The model under review builds one solid part; all positions refer to its coordinate system, in mm. Face numbers are marked on the shaded views. A direction names the side the tool comes from. Give positions to 0.01 mm unless a question says otherwise; leave off trailing zeros. Order: outer loops, then holes, each group sorted by start corner. A loop starts at its lowest first (then second) coordinate and runs counter-clockwise, first axis right, second up. Notation, with made-up numbers: (12, 74) - (69, 74) arc R21 cw to (69, 107) - close; hole circle Ø9 at (24, -38). An arc over 180 degrees is marked (long way). Use CSV: the item, a comma, the result in double quotes.
```python
from build123d import *

# Parameters (mm, degrees)
F1_DEPTH  = 44
F3_DEPTH  = 45.2
F4_DEPTH  = 52
F5_R      = 4
F6_DEPTH  = 57.3
F7_R      = 7.25
F8_DEPTH  = 25
F9_R      = 3
F10_R     = 3
F11_R     = 3
F12_R     = 3
F14_DEPTH = 25
F15_DEPTH = 25
F17_DEPTH = 25
F18_DEPTH = 25
F19_DEPTH = 25
F21_DEPTH = 25


with BuildPart() as f1:
    # F0 (on Front) → F1 (new body)
    with BuildSketch(Plane.XZ):
        Polygon((-81.5560135724, 81.1066666667), (-81.5560135724, 0), (-79.1760135724, 0), (-79.1760135724, 78.7266666667), (-49.1760135724, 78.7266666667), (-49.1760135724, 0), (-46.7960135724, 0), (-46.7960135724, 81.1066666667), align=None)
    extrude(amount=F1_DEPTH)

    # F2 (on face) → F3 (cut)
    with BuildSketch(Plane.YZ.offset(-46.7960135724)):
        with BuildLine():
            ThreePointArc((-10.0000000069, 0), (-15.8590620568, 1.8962112679), (-19.4961202132, 6.8657216307))
            Line((-19.4961202132, 6.8657216307), (-44, 81.1066666667))
            Line((-44, 81.1066666667), (-44, 0))
            Line((-44, 0), (-10.0000000069, 0))
        make_face()
    extrude(amount=-F3_DEPTH, mode=Mode.SUBTRACT)

    # F2 (on face) → F4 (cut)
    with BuildSketch(Plane.YZ.offset(-46.7960135724)):
        with BuildLine():
            ThreePointArc((0, 10.0000000432), (-2.9289321753, 2.928932201), (-10.0000000069, 0))
            Line((-10.0000000069, 0), (0, 0))
            Line((0, 0), (0, 10.0000000432))
        make_face()
    extrude(amount=-F4_DEPTH, mode=Mode.SUBTRACT)

    # F5 (on face) → F6 (cut)
    with BuildSketch(Plane(origin=(-81.5560135724, 0, 0), x_dir=(0, -1, 0), z_dir=(-1, 0, 0))):
        with Locations((10, 10)):
            Circle(F5_R)
    extrude(amount=-F6_DEPTH, mode=Mode.SUBTRACT)

    # F7 (on face) → F8 (cut)
    with BuildSketch(Plane.XY.offset(81.1066666667)):
        with Locations((-64.1760135724, -22)):
            Circle(F7_R)
    extrude(amount=-F8_DEPTH, mode=Mode.SUBTRACT)

    # F9
    f9_edges = [f1.edges().sort_by_distance(p)[0] for p in [
        (-81.556014, -22, 81.106667),
    ]]
    fillet(f9_edges, radius=F9_R)

    # F10
    f10_edges = [f1.edges().sort_by_distance(p)[0] for p in [
        (-46.796014, -22, 81.106667),
    ]]
    fillet(f10_edges, radius=F10_R)

    # F11
    f11_edges = [f1.edges().sort_by_distance(p)[0] for p in [
        (-49.176014, -21.60723, 78.726667),
    ]]
    fillet(f11_edges, radius=F11_R)

    # F12
    f12_edges = [f1.edges().sort_by_distance(p)[0] for p in [
        (-79.176014, -21.60723, 78.726667),
    ]]
    fillet(f12_edges, radius=F12_R)

    # F13 (on face) → F14 (cut)
    with BuildSketch(Plane.YZ.offset(-46.7960135724)):
        Polygon((-11.25, 16), (-11.25, 14), (-11.25, 13.495109044), (-10, 13.5341417044), (-8.75, 13.5731743649), (-8.75, 14), (-8.75, 16), align=None)
    extrude(amount=-F14_DEPTH, mode=Mode.SUBTRACT)

    # F13 (on face) → F15 (cut)
    with BuildSketch(Plane.YZ.offset(-46.7960135724)):
        Polygon((-11.25, 16), (-11.25, 14), (-11.25, 13.495109044), (-10, 13.5341417044), (-8.75, 13.5731743649), (-8.75, 14), (-8.75, 16), align=None)
    extrude(amount=-F15_DEPTH, mode=Mode.SUBTRACT)

    # F13 (on face) → F18 (cut)
    with BuildSketch(Plane.YZ.offset(-46.7960135724)):
        Polygon((-11.25, 16), (-11.25, 14), (-11.25, 13.495109044), (-10, 13.5341417044), (-8.75, 13.5731743649), (-8.75, 14), (-8.75, 16), align=None)
    extrude(amount=-F18_DEPTH, mode=Mode.SUBTRACT)

    # F13 (on face) → F21 (cut)
    with BuildSketch(Plane.YZ.offset(-46.7960135724)):
        Polygon((-11.25, 16), (-11.25, 14), (-11.25, 13.495109044), (-10, 13.5341417044), (-8.75, 13.5731743649), (-8.75, 14), (-8.75, 16), align=None)
    extrude(amount=-F21_DEPTH, mode=Mode.SUBTRACT)


with BuildPart() as f17:
    # F5 (on face) → F17 (new body)
    with BuildSketch(Plane(origin=(-81.5560135724, 0, 0), x_dir=(0, -1, 0), z_dir=(-1, 0, 0))):
        with Locations((10, 10)):
            Circle(F5_R)
    extrude(amount=F17_DEPTH)

    # F19 (cut): a face of the model
    f19_faces = [f17.faces().sort_by_distance(p)[0] for p in [
        (-106.5560135724, -10, 10),
    ]]
    extrude(f19_faces, amount=-F19_DEPTH, mode=Mode.SUBTRACT)


solid = f1.part
```
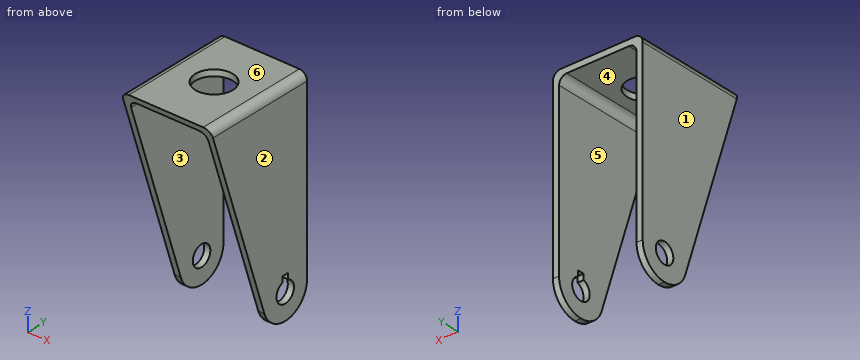
Item 1: Take a section at A-A, the plane z = 67. Give the boundary of the cut face in (x, y), and give its area (3 significant figures).
Results list:
outline,"(-81.56, -39.34) - (-79.18, -39.34) - (-79.18, 0) - (-81.56, 0) - close; (-49.18, -39.34) - (-46.8, -39.34) - (-46.8, 0) - (-49.18, 0) - close"
area,"187 mm2"
Item 2: Take a section at D-D, the plane y = -38. Give the boundary of the cut face in (x, z), and give its area (3 significant figures).
Results list:
outline,"(-81.56, 62.93) - (-79.18, 62.93) - (-79.18, 75.73) arc R3 cw to (-76.18, 78.73) - (-52.18, 78.73) arc R3 cw to (-49.18, 75.73) - (-49.18, 62.93) - (-46.8, 62.93) - (-46.8, 78.11) arc R3 ccw to (-49.8, 81.11) - (-78.56, 81.11) arc R3 ccw to (-81.56, 78.11) - close"
area,"158 mm2"
Item 3: Clearance check with flat-ended pins moving along their axes: pin 1 (1 mm diameter, centred on x = -77, z = 61.5, fed in from -Y); pin 2 (1.8 mm diameter, centred on x = -48.5, z = 15, fed in from -Y); pin 3 (6 mm diameter, centred on x = -63.5, y = -34.5, fed in from -Z). State where each tip first meets the part, or that it passes through.
Results list:
pin 1,"passes through"
pin 2,"stops at y = -22.48"
pin 3,"stops at z = 78.73"
Item 4: Tool access review of the marked faces 5 and 6: name each direction out of +Z, -Z, +X, -X, +Y, -Y from which nothing blocks a thin tool from reaching the whole face with its end or side.
Results list:
face 5,"-Z, +Y, -Y"
face 6,"+Z, +X, -X, +Y, -Y"
Item 5: Wall thickness on L1, parallel to X at y = -29, z = 68.5; L2, parallel to Z at x = -72, y = -40; L3, parallel to Z at x = -81.05, y = -10: over which ranges is each line inside the solid? List them lowest first.
Results list:
L1,"x = -81.56 to -79.18, -49.18 to -46.8"
L2,"z = 78.73 to 81.11"
L3,"z = 0 to 6, 14 to 79.77"
Item 6: Take a section at B-B, the plane x = -69. Give the boundary of the cut face in (y, z), and give its area (3 significant figures).
Results list:
outline,"(-44, 81.11) - (-43.21, 78.73) - (-27.41, 78.73) - (-27.41, 81.11) - close; (-16.59, 78.73) - (0, 78.73) - (0, 81.11) - (-16.59, 81.11) - close"
area,"78.0 mm2"
Item 7: Mouldability with a two-part tool opening along X and no side actions: class the marked faces 1, 2, 3 and 4 as pulls with the +X half, pulls with the -X half, needs draft (parallel to the pull), parting line crosses it, or undercut.
Results list:
face 1,"pulls with the -X half"
face 2,"pulls with the +X half"
face 3,"undercut"
face 4,"undercut"
Item 8: Take a section at C-C, the plane y = -22. Give the boundary of the cut face in (x, z), and give its area (3 significant figures).
Results list:
outline,"(-81.56, 14.45) - (-79.18, 14.45) - (-79.18, 75.73) arc R3 cw to (-76.18, 78.73) - (-71.43, 78.73) - (-71.43, 81.11) - (-78.56, 81.11) arc R3 ccw to (-81.56, 78.11) - close; (-56.93, 78.73) - (-52.18, 78.73) arc R3 cw to (-49.18, 75.73) - (-49.18, 14.45) - (-46.8, 14.45) - (-46.8, 78.11) arc R3 ccw to (-49.8, 81.11) - (-56.93, 81.11) - close"
area,"354 mm2"
